Job drawing, mm, ordinate dimensions from the low corner. One solid piece. Round coordinates to 2 decimals unless told otherwise and drop trailing zeros. Write each loop counter-clockwise with the first axis right and the second up, starting at its lowest first coordinate (ties: lowest second). Pieces come first, ordered by that corner, then holes. Notation, with made-up numbers: (39.5, -24.75) -> (68.5, -24.75) arc R17 cw to (68.5, 3.25) -> close; hole circle Ø2 at (29, -20.5). An arc over 180 degrees is marked (long way). Use CSV: the item, a comma, the result in double quotes. Start each with the question number.
(1) Drop a flat-ended pin along its axis: pin 1 (4.5 mm diameter, centred on x = 12.7, y = 25.4, fed in from +Z). Give the stop position or say it passes through.
(2) Probe line 1 (X direction, y = 25.4, z = 0.65) (1 decimal); line 2 (X direction, y = 10, z = 0.6) (1 decimal); line 3 (Y direction, x = 15.5, z = 0.35) (1 decimal). List the from-to ranges inside material, lowest first. Write a range as [from, to].
(3) Saw through at C-C (y = 35). Give the cut face in (x, z) (1 decimal).
(4) Saw through at B-B (z = 1.55). Count the separate pieces of the cut face and the enclosed holes in it, plus the area to 3 significant figures.
(5) Saw through at A-A (x = 31.75). Give the cut face in (y, z) (1 decimal).
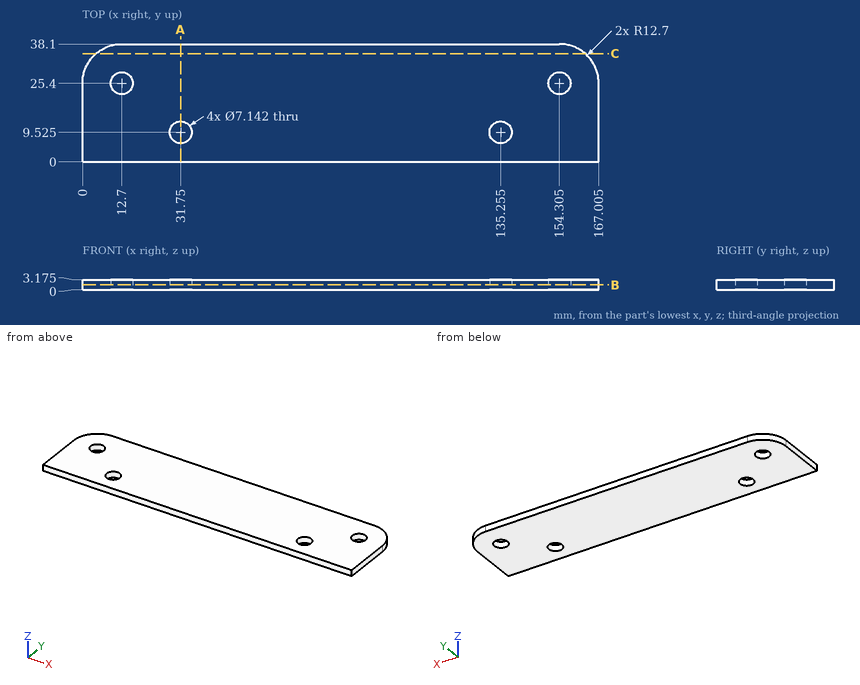
Answers:
1,pin 1,"passes through"
2,line 1,"x = [0, 9.1], [16.3, 150.7], [157.9, 167]"
2,line 2,"x = [0, 28.2], [35.3, 131.7], [138.8, 167]"
2,line 3,"y = [0, 23.2], [27.6, 38.1]"
3,outline,"(4.4, 0) -> (162.6, 0) -> (162.6, 3.2) -> (4.4, 3.2) -> close"
4,separate pieces,"1"
4,enclosed holes,"4"
4,area,"6,130 mm²"
5,outline,"(0, 0) -> (6, 0) -> (6, 3.2) -> (0, 3.2) -> close; (13.1, 0) -> (38.1, 0) -> (38.1, 3.2) -> (13.1, 3.2) -> close"
